```python
from build123d import *

# Parameters (mm, degrees)
F1_DEPTH  = 22
F3_R      = 11.25
F4_DEPTH  = 16
F5_DEPTH  = 18
F6_R      = 4.75
F7_DEPTH  = 4
F8_W      = 3
F8_H      = 2
F9_DEPTH  = 22
F11_DEPTH = 15
F12_R     = 11.25
F13_DEPTH = 15
F14_R     = 1.85
F15_DEPTH = 50.8
F17_DEPTH = 9.8


# Not quite as in the source:
# - a feature names something its author has since deleted; it is built from what else it names


with BuildPart() as f1:
    # F0 (on Top) → F1 (new body)
    with BuildSketch(Plane.XY):
        with BuildLine():
            ThreePointArc((1.21e-08, -14), (9.8994949409, -9.8994949323), (14, 0))
            ThreePointArc((14, 0), (9.8994949202, 9.899494953), (-4.65e-08, 14))
            ThreePointArc((-4.65e-08, 14), (-14, -2.93e-08), (1.21e-08, -14))
        make_face()
        with BuildLine():
            ThreePointArc((-4.65e-08, 14), (9.8994949202, 9.899494953), (14, 0))
            ThreePointArc((14, 0), (9.8994949409, -9.8994949323), (1.21e-08, -14))
            Line((1.21e-08, -14), (42, -14))
            Line((42, -14), (42, 14))
            Line((42, 14), (-4.65e-08, 14))
        make_face()
        with BuildLine():
            ThreePointArc((1.21e-08, -14), (-14, -2.93e-08), (-4.65e-08, 14))
            Line((-4.65e-08, 14), (-42, 14))
            Line((-42, 14), (-42, -14))
            Line((-42, -14), (1.21e-08, -14))
        make_face()
    extrude(amount=F1_DEPTH)

    # F3 (on face) → F4 (cut)
    with BuildSketch(Plane.XY.offset(22)):
        Circle(F3_R)
    extrude(amount=-F4_DEPTH, mode=Mode.SUBTRACT)

    # F2 (on face) → F5 (cut)
    with BuildSketch(Plane.XY.offset(22)):
        with BuildLine():
            Line((-6, 3.8887658711), (-6, -3.8887658711))
            ThreePointArc((-6, -3.8887658711), (0, -7.15), (6, -3.8887658711))
            Line((6, -3.8887658711), (6, 3.8887658711))
            ThreePointArc((6, 3.8887658711), (0, 7.15), (-6, 3.8887658711))
        make_face()
    extrude(amount=-F5_DEPTH, mode=Mode.SUBTRACT)

    # F6 (on face) → F7 (cut)
    with BuildSketch(Plane.XY.offset(4)):
        Circle(F6_R)
    extrude(amount=-F7_DEPTH, mode=Mode.SUBTRACT)

    # F8 (on face) → F9 (cut)
    with BuildSketch(Plane.XY.offset(22)):
        with Locations((-26.5, 11)):
            Rectangle(F8_W, F8_H)
        with Locations((-23.5, 11)):
            Rectangle(F8_W, F8_H)
        with Locations((-23.5, -11)):
            Rectangle(F8_W, F8_H)
        with Locations((-26.5, -11)):
            Rectangle(F8_W, F8_H)
        with Locations((23.5, 11)):
            Rectangle(F8_W, F8_H)
        with Locations((26.5, 11)):
            Rectangle(F8_W, F8_H)
        with Locations((26.5, -11)):
            Rectangle(F8_W, F8_H)
        with Locations((23.5, -11)):
            Rectangle(F8_W, F8_H)
    extrude(amount=-F9_DEPTH, mode=Mode.SUBTRACT)

    # F10 (on face) → F11 (join)
    with BuildSketch(Plane.XY.offset(22)):
        Polygon((-21.25, -14), (21.25, -14), (21.25, 0), (21.25, 14), (-21.25, 14), align=None)
    extrude(amount=F11_DEPTH)

    # F12 (on face) → F13 (cut)
    with BuildSketch(Plane.XY.offset(37)):
        Circle(F12_R)
    extrude(amount=-F13_DEPTH, mode=Mode.SUBTRACT)

    # F14 (on face) → F15 (cut)
    with BuildSketch(Plane.YZ.offset(21.25)):
        with Locations((0, 29.2573869228)):
            Circle(F14_R)
    extrude(amount=-F15_DEPTH, mode=Mode.SUBTRACT)

    # F16 (on face) → F17 (cut)
    with BuildSketch(Plane.XY.offset(37)):
        Polygon((-14.25, -4), (-14.25, 4), (-17.75, 4), (-17.75, 1.1981789721), (-17.75, -4), align=None)
        Polygon((14.25, -4), (17.75, -4), (17.75, 0), (17.75, 4), (14.25, 4), align=None)
    extrude(amount=-F17_DEPTH, mode=Mode.SUBTRACT)


solid = f1.part
```
Work out the finished part from the listing and answer in its coordinate system (mm). A direction names the side the tool comes from. Give positions to 0.01 mm unless a question says otherwise; leave off trailing zeros. Order: outer loops, then holes, each group sorted by start corner. A loop starts at its lowest first (then second) coordinate and runs counter-clockwise, first axis right, second up.
1. For faces 5 (the flat face through (-21.25, 3, 29)), 6 (the flat face through (31, 0, 22)), 7 (the flat face through (-28, 11, 11)), 8 (the flat face through (-16, 4, 32)), 9 (the flat face through (-1, -14, 14)), determine the directions among +Z, -Z, +X, -X, +Y, -Y from which every point of the face is accessible in a straight line to the end or side of a thin tool.
Result sheet:
face 5: +Z, -X, +Y, -Y
face 6: +Z, +X, +Y, -Y
face 7: +Z, -Z
face 8: +Z
face 9: +Z, -Z, +X, -X, -Y
2. Section A-A, the plane z = 33.5 is taken. Determine the outline of the cut face in (x, y).
Result sheet:
outline: (-21.25, -14) - (21.25, -14) - (21.25, 14) - (-21.25, 14) - close; hole (-17.75, -4) - (-14.25, -4) - (-14.25, 4) - (-17.75, 4) - close; hole circle Ø22.5 at (0, 0); hole (14.25, -4) - (17.75, -4) - (17.75, 4) - (14.25, 4) - close
3. Straight lines are drawn through the part: L1, parallel to Y at x = 26.5, z = 16; L2, parallel to Z at x = -20.45, y = 0; L3, parallel to Y at x = 0, z = 2.1. For each, find the intervals that lie inside material, in ascending order.
Result sheet:
L1: y = -14 to -12, -10 to 10, 12 to 14
L2: z = 0 to 27.41, 31.11 to 37
L3: y = -14 to -4.75, 4.75 to 14
4. The mould has two halves that part along X. Classify faces 1 (the flat face through (-32, 0, 22)), 2 (the flat face through (17.75, 0, 32)), 3 (the flat face through (-42, 0, 11)), 4 (the flat face through (28, 11, 11)): released by +X, released by -X, zero draft, split by the parting line, or undercut.
Result sheet:
face 1: zero draft
face 2: undercut
face 3: released by -X
face 4: undercut
5. Section D-D, the plane y = 8.75 is taken. Determine the outline of the cut face in (x, z), and give its area (3 significant figures).
Result sheet:
outline: (-42, 0) - (42, 0) - (42, 22) - (21.25, 22) - (21.25, 37) - (7.07, 37) - (7.07, 6) - (-7.07, 6) - (-7.07, 37) - (-21.25, 37) - (-21.25, 22) - (-42, 22) - close
area: 2,050 mm2
6. Each of these flat-tipped pins is pushed along its axis until it touches: P1, Ø4.5, axis at y = 6, z = 32.5, coming from the -X side; P2, Ø6, axis at y = 0, z = 29.26, coming from the +X side; P3, Ø3, axis at x = -30, z = 24, coming from the +Y side. Where does it stop, or does it pass through?
Result sheet:
P1: stops at x = -21.25
P2: stops at x = 21.25
P3: passes through
7. Section B-B, the plane x = 0 is taken. Determine the outline of the cut face in (y, z).
Result sheet:
outline: (-14, 0) - (-4.75, 0) - (-4.75, 4) - (-7.15, 4) - (-7.15, 6) - (-11.25, 6) - (-11.25, 37) - (-14, 37) - close; (4.75, 0) - (14, 0) - (14, 37) - (11.25, 37) - (11.25, 6) - (7.15, 6) - (7.15, 4) - (4.75, 4) - close
8. Section C-C, the plane z = 8 is taken. Determine the outline of the cut face in (x, y).
Result sheet:
outline: (-42, -14) - (42, -14) - (42, 14) - (-42, 14) - close; hole (-28, -12) - (-22, -12) - (-22, -10) - (-28, -10) - close; hole (-28, 10) - (-22, 10) - (-22, 12) - (-28, 12) - close; hole circle Ø22.5 at (0, 0); hole (22, -12) - (28, -12) - (28, -10) - (22, -10) - close; hole (22, 10) - (28, 10) - (28, 12) - (22, 12) - close
